For this review, use the dimensioned drawing (mm, ordinates from the lowest corner) and the shaded views. Round coordinates to 2 decimals unless told otherwise and drop trailing zeros. Order: outer loops, then holes, each group sorted by start corner. A loop starts at its lowest first (then second) coordinate and runs counter-clockwise, first axis right, second up. Notation, with made-up numbers: (-38.75, 24) - (10.25, 24) arc R16 cw to (10.25, 55) - close; hole circle Ø6 at (1, 84.5). An arc over 180 degrees is marked (long way). Write each question's results on one line, items separated by ' | '. Start each with the question number.
(1) Take a section at C-C, the plane y = 15.5. Give the boundary of the cut face in (x, z).
(2) Take a section at B-B, the plane x = 3.1. Give the boundary of the cut face in (y, z).
(3) Draft analysis for pull direction X (two halves, no side actions). For the marked faces 1, 2 and 3, state which applies: pulls with the +X half, pulls with the -X half, needs draft (parallel to the pull), parting line crosses it, or undercut.
(4) For L1, parallel to Y at x = 38.1, z = 1.4; L2, parallel to X at y = 53, z = 1.3 (1 decimal); L3, parallel to X at y = 30, z = 0.35, list the stretches that pass through material, from the lowest coordinate up. Write a range as from..to.
(5) Take a section at A-A, the plane y = 28.1. Give the boundary of the cut face in (x, z) (1 decimal).
(6) Insertion check: pin 1 Ø5 at (x, y) = (38.1, 73.1) entering from -Z; pin 2 Ø3 at (y, z) = (47.5, 3.5) entering from +X; pin 3 Ø1 at (y, z) = (42, 3) entering from +X; pin 4 Ø2 at (y, z) = (67.5, 4) entering from +X. Each pin has a flat end and moves straight along its axis. Give the tip position at first contact, or say it passes through.
(7) Take a section at D-D, the plane z = 1.15. Give the number of separate pieces and of enclosed holes in the cut face, plus the area to 3 significant figures.
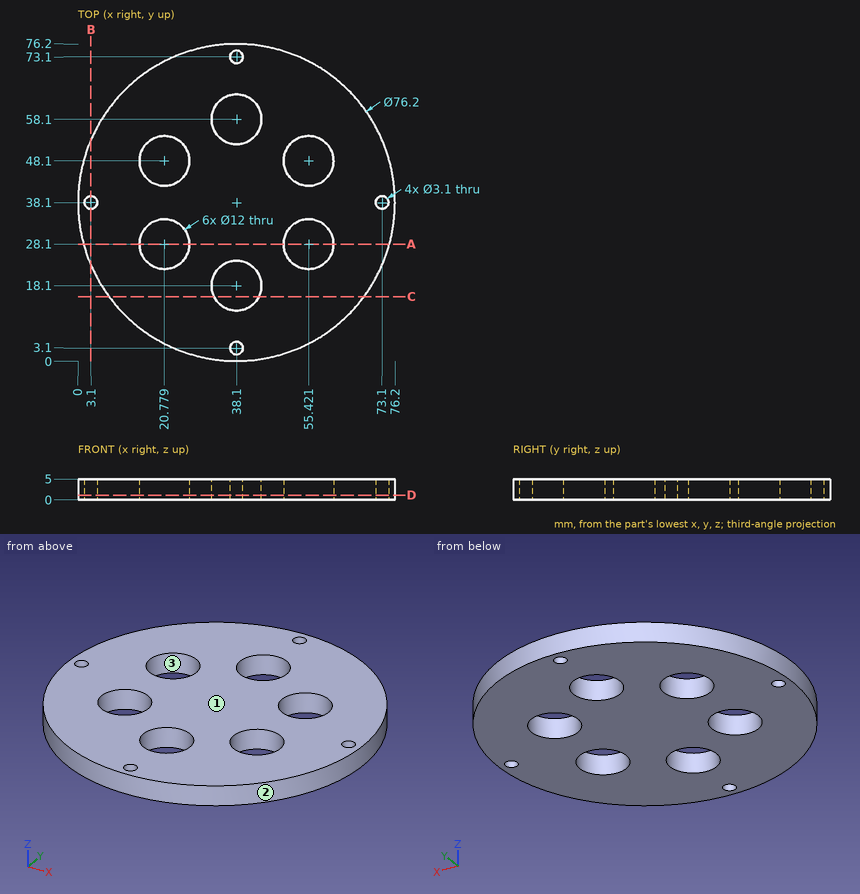
Results below:
1) outline: (7.43, 0) - (32.69, 0) - (32.69, 5) - (7.43, 5) - close; (43.51, 0) - (68.77, 0) - (68.77, 5) - (43.51, 5) - close
2) outline: (23.05, 0) - (36.55, 0) - (36.55, 5) - (23.05, 5) - close; (39.65, 0) - (53.15, 0) - (53.15, 5) - (39.65, 5) - close
3) face 1: needs draft | face 2: parting line crosses it | face 3: undercut
4) L1: y = 0..1.55, 4.65..12.1, 24.1..52.1, 64.1..71.55, 74.65..76.2 | L2: x = 3..17.3, 24.2..34.9, 41.3..52, 58.9..73.2 | L3: x = 0.87..15.09, 26.47..49.73, 61.11..75.33
5) outline: (1.3, 0) - (14.8, 0) - (14.8, 5) - (1.3, 5) - close; (26.8, 0) - (49.4, 0) - (49.4, 5) - (26.8, 5) - close; (61.4, 0) - (74.9, 0) - (74.9, 5) - (61.4, 5) - close
6) pin 1: stops at z = 0 | pin 2: stops at x = 75.37 | pin 3: stops at x = 76.05 | pin 4: stops at x = 63.5
7) separate pieces: 1 | enclosed holes: 10 | area: 3,850 mm^2
